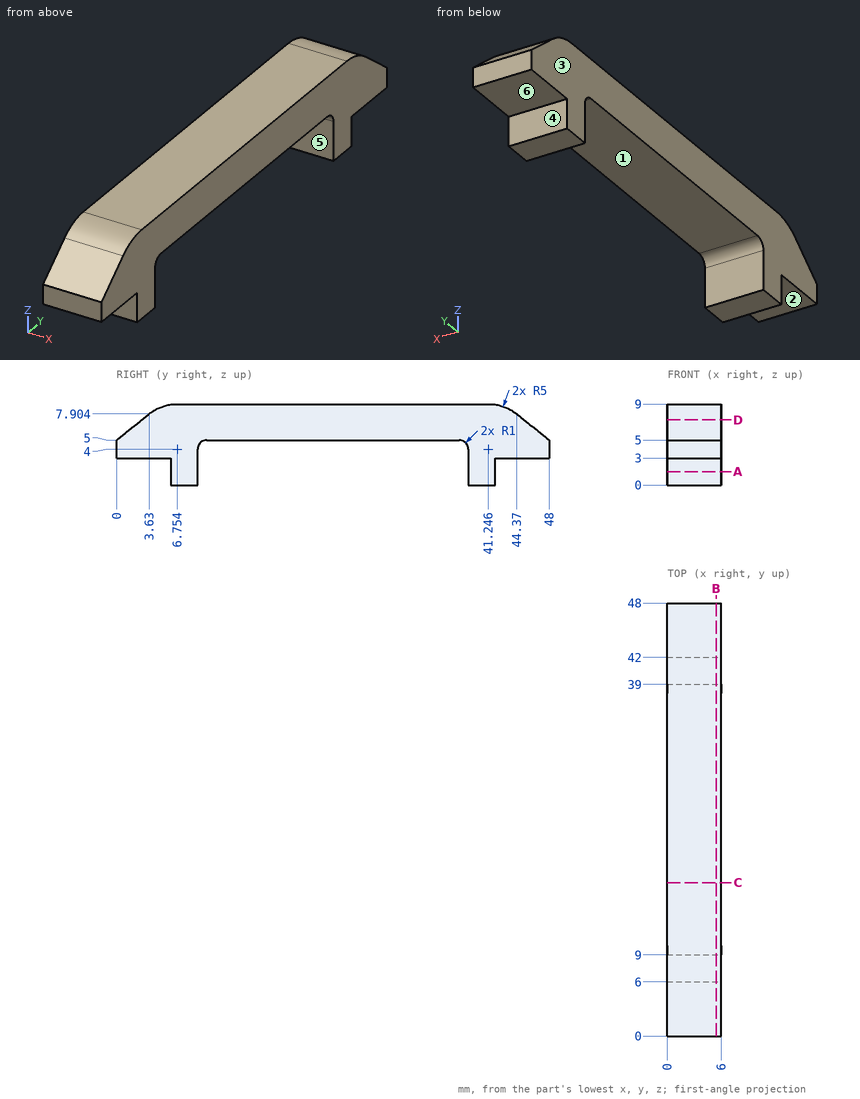
Check sheet for the drawn part. Datum: minimum x, y, z corner. Units: mm. A direction names the side the tool comes from. Coordinates: 2 decimals unless noted, no trailing zeros. Write each loop counter-clockwise with the first axis right and the second up, starting at its lowest first coordinate (ties: lowest second). Pieces come first, ordered by that corner, then holes. Notation, with made-up numbers: (67, 79) - (113, 79) arc R26 ccw to (113, 112) - close; hole circle Ø8 at (20, 30.25). An arc over 180 degrees is marked (long way). Answer as a JSON object with one key per item and string values.
(1) Tool access check on the marked faces 1, 2 and 3. Record the directions out of +Z, -Z, +X, -X, +Y, -Y that give a thin tool (end or side, any length) a straight path to the whole face; none if there is none.
Report:
{"face 1": "-Z, +X, -X", "face 2": "-Z, +X, -X, -Y", "face 3": "+Z, -Z, -X, +Y, -Y"}
(2) Mould release check, pull along Y, two halves, no side actions. Record for the marked faces 4, 5 and 6: pulls with the +Y half, pulls with the -Y half, needs draft (parallel to the pull), parting line crosses it, or undercut.
Report:
{"face 4": "pulls with the +Y half", "face 5": "undercut", "face 6": "needs draft"}
(3) Cross-section at D-D on z = 7.25. Record the cut outline in (x, y), plus the area to 3 significant figures.
Report:
{"outline": "(0, 2.81) - (6, 2.81) - (6, 45.19) - (0, 45.19) - close", "area": "254 mm^2"}
(4) Cross-section at B-B on x = 5.4. Record the cut outline in (y, z) (1 decimal).
Report:
{"outline": "(0, 3) - (6, 3) - (6, 0) - (9, 0) - (9, 4) arc R1 cw to (10, 5) - (38, 5) arc R1 cw to (39, 4) - (39, 0) - (42, 0) - (42, 3) - (48, 3) - (48, 5) - (44.4, 7.9) arc R5 ccw to (41.2, 9) - (6.8, 9) arc R5 ccw to (3.6, 7.9) - (0, 5) - close"}
(5) Thickness scan on line 1 along Y through (x, z) = (4.65, 2.5); line 2 along Y through (x, z) = (5.25, 3.25); line 3 along Z through (x, y) = (2.15, 23). Record the ranges inside material, lowest first.
Report:
{"line 1": "6 to 9, 39 to 42", "line 2": "0 to 9, 39 to 48", "line 3": "5 to 9"}
(6) Cross-section at C-C on y = 17. Record the cut outline in (x, z).
Report:
{"outline": "(0, 5) - (6, 5) - (6, 9) - (0, 9) - close"}
(7) Cross-section at A-A on z = 1.5. Record the cut outline in (x, y), plus the area to 3 significant figures.
Report:
{"outline": "(0, 6) - (6, 6) - (6, 9) - (0, 9) - close; (0, 39) - (6, 39) - (6, 42) - (0, 42) - close", "area": "36.0 mm^2"}
(8) Gauge pin test, flat ends, axial feed: pin 1 Ø1.5 at (x, z) = (3, 1.5) entering from -Y; pin 2 Ø1 at (x, y) = (3, 10.5) entering from -Z; pin 3 Ø3 at (x, z) = (4, 6) entering from -Y; pin 4 Ø1.8 at (x, y) = (4, 3.5) entering from -Z. Record the tip position at first contact, or that the pin passes through.
Report:
{"pin 1": "y = 6", "pin 2": "z = 5", "pin 3": "y = 0", "pin 4": "z = 3"}
